from build123d import *

# Parameters (mm, degrees)
F1_DEPTH = 20
F2_R     = 4
F3_DEPTH = 20.001


with BuildPart() as f1:
    # F0 (on Top) → F1 (new body)
    with BuildSketch(Plane.XY):
        Polygon((-50, 0), (0, 0), (50, 0), (50, 20), (15, 20), (15, 100), (0, 100), (-15, 100), (-15, 20), (-50, 20), align=None)
    extrude(amount=F1_DEPTH)

    # F2 (on face) → F3 (cut, through all)
    with BuildSketch(Plane.XY.offset(20)):
        with Locations((0, 80)):
            Circle(F2_R)
    extrude(amount=-F3_DEPTH, mode=Mode.SUBTRACT)


solid = f1.part
For this review, take the finished solid that the model builds, in its own axes (mm). A direction names the side the tool comes from. Give positions to 0.01 mm unless a question says otherwise; leave off trailing zeros. Loops run counter-clockwise (first coordinate to the right, second up) from the corner with the lowest first, then second, coordinate; pieces in that order, holes last. Notation, with made-up numbers: M 38.5,46.5 L 97.5,46.5 A22 ccw 97.5,55.5 Z; hole C 87.25,89.5 d8. An arc over 180 degrees is marked long. Answer as a JSON object with one key per item and string values. Group by question number.
Q1. Add section A-A on y = 80. Give the boundary of the cut face in (x, z), and give its area (3 significant figures).
Q2. For probe 1 along X at (y, z) = (22, 11.5); probe 2 along Y at (x, z) = (40, 15.5); probe 3 along X at (y, z) = (82, 14.5), list the stretches that pass through material, from the lowest coordinate up. Write a range as [from, to].
Q3. Add section B-B on z = 11.25. Give the boundary of the cut face in (x, y).
Q4. Tool access review of faces 5 (the flat face through (0, 100, 10)), 6 (the flat face through (33, 20, 10)), 7 (the flat face through (-15, 61, 10)): name each direction out of +Z, -Z, +X, -X, +Y, -Y from which nothing blocks a thin tool from reaching the whole face with its end or side.
Q5. Mouldability with a two-part tool opening along X and no side actions: class faces 1 (the flat face through (-1, 40, 0)), 2 (the flat face through (-50, 10, 10)), 3 (the flat face through (50, 10, 10)), 4 (the cylindrical face through (-0.867, 76.095, 10.14)) as +X half, -X half, draft (parallel to the pull), parting line (faces both ways), or undercut.
Q6. Add section D-D on y = 52. Give the boundary of the cut face in (x, z), and give its area (3 significant figures).
Q7. Insertion check: P1, Ø6, axis at y = 53.5, z = 9, coming from the +X side; P2, Ø6.5, axis at x = 0, y = 80, coming from the -Z side; P3, Ø6, axis at x = -32, z = 10, coming from the +Y side; P4, Ø6, axis at y = 45.5, z = 13, coming from the -X side. Each pin has a flat end and moves straight along its axis. Give the tip position at first contact, or say it passes through.
Q8. Add section C-C on x = 0. Give the boundary of the cut face in (y, z), and give its area (3 significant figures).
Checked values:
{
 "1": {"outline": "M -15,0 L -4,0 L -4,20 L -15,20 Z; M 4,0 L 15,0 L 15,20 L 4,20 Z", "area": "440 mm²"},
 "2": {"probe 1": "[-15, 15]", "probe 2": "[0, 20]", "probe 3": "[-15, -3.46], [3.46, 15]"},
 "3": {"outline": "M -50,0 L 50,0 L 50,20 L 15,20 L 15,100 L -15,100 L -15,20 L -50,20 Z; hole C 0,80 d8"},
 "4": {"face 5": "+Z, -Z, +X, -X, +Y", "face 6": "+Z, -Z, +X, +Y", "face 7": "+Z, -Z, -X, +Y"},
 "5": {"face 1": "draft", "face 2": "-X half", "face 3": "+X half", "face 4": "undercut"},
 "6": {"outline": "M -15,0 L 15,0 L 15,20 L -15,20 Z", "area": "600 mm²"},
 "7": {"P1": "x = 15", "P2": "through", "P3": "y = 20", "P4": "x = -15"},
 "8": {"outline": "M 0,0 L 76,0 L 76,20 L 0,20 Z; M 84,0 L 100,0 L 100,20 L 84,20 Z", "area": "1,840 mm²"}
}
